```python
from build123d import *

# Parameters (mm, degrees)
SKETCH_R   = 2
SKETCH_R_2 = 1.5
SKETCH_W   = 41.9
SKETCH_H   = 20
PAD_DEPTH  = 3


with BuildPart() as part:
    # Sketch → Pad (new body)
    with BuildSketch(Plane.XY):
        Polygon((0, 88.15), (14, 88.15), (14, 76.75), (25.4, 76.75), (25.4, 88.15), (58.3, 88.15), (58.3, 76.75), (69.7, 76.75), (69.7, 88.15), (84, 88.15), (84, 11.4), (78.3, 11.4), (78.3, 0), (11.4, 0), (11.4, 11.4), (0, 11.4), align=None)
        with Locations((16.74, 71.15)):
            Circle(SKETCH_R, mode=Mode.SUBTRACT)
        with Locations((33.48, 71.15)):
            Circle(SKETCH_R, mode=Mode.SUBTRACT)
        with Locations((50.22, 71.15)):
            Circle(SKETCH_R, mode=Mode.SUBTRACT)
        with Locations((66.96, 71.15)):
            Circle(SKETCH_R, mode=Mode.SUBTRACT)
        with Locations((73, 15)):
            Circle(SKETCH_R_2, mode=Mode.SUBTRACT)
        with Locations((9, 57.15)):
            Circle(SKETCH_R_2, mode=Mode.SUBTRACT)
        with Locations((9, 37.15)):
            Circle(SKETCH_R_2, mode=Mode.SUBTRACT)
        with Locations((37.35, 15)):
            Rectangle(SKETCH_W, SKETCH_H, mode=Mode.SUBTRACT)
    pad = extrude(amount=PAD_DEPTH)

    # Mirrored: Pad across face of Pad
    add(pad.mirror(Plane(origin=(84, 49.775, 1.5), x_dir=(0, 1, 0), z_dir=(1, 0, 0))))


solid = part.part
```
The model under review builds one solid part; all positions refer to its coordinate system, in mm. A direction names the side the tool comes from. Round coordinates to 2 decimals unless told otherwise and drop trailing zeros. Loops run counter-clockwise (first coordinate to the right, second up) from the corner with the lowest first, then second, coordinate; pieces in that order, holes last.
Item 1: Take a section at A-A (y = 80). Write out the cut boundary in (x, z), then the cut area to 3 significant figures.
Determined:
outline: (0, 0) - (14, 0) - (14, 3) - (0, 3) - close; (25.4, 0) - (58.3, 0) - (58.3, 3) - (25.4, 3) - close; (69.7, 0) - (98.3, 0) - (98.3, 3) - (69.7, 3) - close; (109.7, 0) - (142.6, 0) - (142.6, 3) - (109.7, 3) - close; (154, 0) - (168, 0) - (168, 3) - (154, 3) - close
area: 367 mm2
Item 2: Take a section at D-D (z = 1.45). Give the number of separate pieces and of enclosed holes in the cut face, then the cut area to 3 significant figures.
Determined:
separate pieces: 1
enclosed holes: 16
area: 12,100 mm2
Item 3: Mouldability with a two-part tool opening along Y and no side actions: class faces 4 (the face through (45, 0, 1)), 5 (the face through (109.7, 15, 1)), 6 (the face through (142.6, 82, 1)) as released by +Y, released by -Y, zero draft, split by the parting line, or undercut.
Determined:
face 4: released by -Y
face 5: undercut
face 6: zero draft
Item 4: Take a section at C-C (x = 112.5). Write out the cut boundary in (y, z), then the cut area to 3 significant figures.
Determined:
outline: (0, 0) - (5, 0) - (5, 3) - (0, 3) - close; (25, 0) - (88.15, 0) - (88.15, 3) - (25, 3) - close
area: 204 mm2
Item 5: For line 1 (Y direction, x = 159, z = 1.05); line 2 (Y direction, x = 16.74, z = 2.35); line 3 (X direction, y = 5.5, z = 0.7), list the stretches that pass through material, from the lowest coordinate up.
Determined:
line 1: y = 11.4 to 35.65, 38.65 to 55.65, 58.65 to 88.15
line 2: y = 0 to 5, 25 to 69.15, 73.15 to 76.75
line 3: x = 11.4 to 16.4, 58.3 to 78.3, 89.7 to 109.7, 151.6 to 156.6
Item 6: For faces 1 (the face through (16.4, 15, 1)), 2 (the face through (84, 11.4, 1)), 3 (the face through (69.7, 82, 1)), list the 3-axis set-ups (+Z, -Z, +X, -X, +Y, -Y) from which the entire face can be reached by the end or side of a thin tool; tool diameter is ignored.
Determined:
face 1: +Z, -Z
face 2: +Z, -Z, -Y
face 3: +Z, -Z, +Y
Item 7: Clearance check with flat-ended pins moving along their axes: pin 1 Ø0.9 at (x, z) = (101.5, 1) entering from +Y; pin 2 Ø1.5 at (y, z) = (4.5, 1) entering from -X; pin 3 Ø0.9 at (y, z) = (4, 1.5) entering from +X. State where each tip first meets the part, or that it passes through.
Determined:
pin 1: stops at y = 76.75
pin 2: stops at x = 11.4
pin 3: stops at x = 156.6
Item 8: Take a section at B-B (x = 50.22). Write out the cut boundary in (y, z).
Determined:
outline: (0, 0) - (5, 0) - (5, 3) - (0, 3) - close; (25, 0) - (69.15, 0) - (69.15, 3) - (25, 3) - close; (73.15, 0) - (88.15, 0) - (88.15, 3) - (73.15, 3) - close
